Geometry: final body of the model. Coordinates: model frame, mm. Give positions to 0.01 mm unless a question says otherwise; leave off trailing zeros. Write each loop counter-clockwise with the first axis right and the second up, starting at its lowest first coordinate (ties: lowest second). Pieces come first, ordered by that corner, then holes. Notation, with made-up numbers: (40, 15.25) -> (88, 15.25) arc R30 cw to (88, 47.25) -> close; hole circle Ø11 at (48, 53). An arc over 180 degrees is marked (long way). Answer as a JSON object with one key per item and string values.
from build123d import *

# Parameters (mm, degrees)
SKETCH005_R  = 2.5
PAD003_DEPTH = 260


with BuildPart() as part:
    # Sketch005 → Pad003 (new body)
    with BuildSketch(Plane.XY):
        with BuildLine():
            Line((-4, -2.585786), (-4, 2.585787))
            Line((-4, 2.585787), (-6.914214, 5.500001))
            Line((-6.914214, 5.500001), (-8, 5.500001))
            Line((-8, 5.500001), (-8, 2.500001))
            Line((-8, 2.500001), (-10, 2.500001))
            Line((-10, 2.500001), (-10, 9.000001))
            ThreePointArc((-9, 10), (-9.707107, 9.707107), (-10, 9.000001))
            Line((-2.5, 10), (-9, 10))
            Line((-2.5, 8), (-2.5, 10))
            Line((-5.5, 8), (-2.5, 8))
            Line((-5.5, 6.914214), (-5.5, 8))
            Line((-2.585786, 4), (-5.5, 6.914214))
            Line((2.585786, 4), (-2.585786, 4))
            Line((2.585786, 4), (5.5, 6.914214))
            Line((5.5, 6.914214), (5.5, 8))
            Line((5.5, 8), (2.5, 8))
            Line((2.5, 8), (2.5, 10))
            Line((2.5, 10), (9, 10))
            ThreePointArc((10, 9.000001), (9.707107, 9.707107), (9, 10))
            Line((10, 2.500001), (10, 9.000001))
            Line((8, 2.500001), (10, 2.500001))
            Line((8, 5.500001), (8, 2.500001))
            Line((6.914214, 5.500001), (8, 5.500001))
            Line((4, 2.585787), (6.914214, 5.500001))
            Line((4, 2.585787), (4, -2.585786))
            Line((4, -2.585786), (6.914214, -5.500001))
            Line((6.914214, -5.500001), (8, -5.500001))
            Line((8, -5.500001), (8, -2.500001))
            Line((8, -2.500001), (10, -2.500001))
            Line((10, -2.500001), (10, -9.000001))
            ThreePointArc((9, -10), (9.707107, -9.707107), (10, -9.000001))
            Line((9, -10), (2.5, -10))
            Line((2.5, -10), (2.5, -8))
            Line((2.5, -8), (5.5, -8))
            Line((5.5, -8), (5.5, -6.914214))
            Line((5.5, -6.914214), (2.585786, -4))
            Line((2.585786, -4), (-2.585786, -4))
            Line((-2.585786, -4), (-5.5, -6.914214))
            Line((-5.5, -6.914214), (-5.5, -8))
            Line((-5.5, -8), (-2.5, -8))
            Line((-2.5, -8), (-2.5, -10))
            Line((-2.5, -10), (-9, -10))
            ThreePointArc((-10, -9.000001), (-9.707107, -9.707107), (-9, -10))
            Line((-10, -2.500001), (-10, -9.000001))
            Line((-8, -2.500001), (-10, -2.500001))
            Line((-8, -5.500001), (-8, -2.500001))
            Line((-6.914214, -5.500001), (-8, -5.500001))
            Line((-4, -2.585786), (-6.914214, -5.500001))
        make_face()
        Circle(SKETCH005_R, mode=Mode.SUBTRACT)
    extrude(amount=PAD003_DEPTH)


solid = part.part
Q1. Mould query, pull axis X, two halves, no side actions, for faces 1 (the flat face through (10, 6, 128)), 2 (the flat face through (-2, 2, 0)), 3 (the cylindrical face through (-0.54, -2.44, 128.18)). Classes: pulls with the +X half, pulls with the -X half, needs draft (parallel to the pull), parting line crosses it, or undercut.
Values:
{"face 1": "pulls with the +X half", "face 2": "needs draft", "face 3": "undercut"}
Q2. Cut plane A-A (x = 0). Return the cut outline in (y, z).
Values:
{"outline": "(-4, 0) -> (-2.5, 0) -> (-2.5, 260) -> (-4, 260) -> close; (2.5, 0) -> (4, 0) -> (4, 260) -> (2.5, 260) -> close"}
Q3. First-contact query: P1, Ø0.6, axis at x = -9.5, z = 175, coming from the +Y side. Flat tip, straight axial feed; report the tip coordinate or a pass-through.
Values:
{"P1": "y = 9.98"}
Q4. Material intervals for L1, parallel to X at y = 7.5, z = 22.5; L2, parallel to X at y = 8.25, z = 30, sorted ascending. Write a range as from..to.
Values:
{"L1": "-10..-5.5, 5.5..10", "L2": "-10..-2.5, 2.5..10"}
